```python
from build123d import *

# Parameters (mm, degrees)
THICKEN1_DEPTH      = 11.6
THICKEN1_START      = 10
THICKEN1_2_DEPTH    = 1.6
SKETCH2_R           = 1
BOSS_EXTRUDE1_DEPTH = 5
SKETCH3_W           = 9
SKETCH3_H           = 4
BOSS_EXTRUDE2_DEPTH = 4.5
CUT_EXTRUDE1_REACH  = 29.786
SKETCH4_RX          = 3.75
SKETCH4_RY          = 2.5
BOSS_EXTRUDE3_START = 7.5
BOSS_EXTRUDE3_DEPTH = 7.5
FILLET1_R           = 0.5
FILLET2_R           = 0.2


# Read off the part's stored shape, not the designer's step: Thicken1
with BuildPart() as part:
    # Thicken1 outline → Thicken1 (new body)
    with BuildSketch(Plane.XY):
        with BuildLine():
            Line((-8.73, -7.62), (8.73, -7.62))
            ThreePointArc((8.73, -7.62), (16.35, 0), (8.73, 7.62))
            Line((8.73, 7.62), (-8.73, 7.62))
            ThreePointArc((-8.73, 7.62), (-16.35, 0), (-8.73, -7.62))
        make_face()
        with BuildLine():
            ThreePointArc((8.73, 6.02), (14.75, 0), (8.73, -6.02))
            Line((8.73, -6.02), (-8.73, -6.02))
            ThreePointArc((-8.73, -6.02), (-14.75, 0), (-8.73, 6.02))
            Line((-8.73, 6.02), (8.73, 6.02))
        make_face(mode=Mode.SUBTRACT)
    extrude(amount=THICKEN1_DEPTH)

    # Thicken1 2 outline → Thicken1 2 (add)
    with BuildSketch(Plane.XY.offset(THICKEN1_START)):
        with BuildLine():
            Line((-8.73, -6.02), (8.73, -6.02))
            ThreePointArc((8.73, -6.02), (14.75, 0), (8.73, 6.02))
            Line((8.73, 6.02), (-8.73, 6.02))
            ThreePointArc((-8.73, 6.02), (-14.75, 0), (-8.73, -6.02))
        make_face()
    extrude(amount=THICKEN1_2_DEPTH)

    # Sketch2 → Boss-Extrude1 (add)
    with BuildSketch(Plane(origin=(0, 0, 10), x_dir=(-1, 0, 0), z_dir=(0, 0, -1))):
        with BuildLine():
            Line((1.6, 6.02), (-1.6, 6.02))
            Line((-1.6, 6.02), (-1.6, 2.537715508))
            ThreePointArc((-1.6, 2.537715508), (-2.537715508, -1.6), (1.6, -2.537715508))
            ThreePointArc((1.6, -2.537715508), (3, 0), (1.6, 2.537715508))
            Line((1.6, 2.537715508), (1.6, 6.02))
        make_face()
        Circle(SKETCH2_R, mode=Mode.SUBTRACT)
    extrude(amount=BOSS_EXTRUDE1_DEPTH)

    # Sketch3 → Boss-Extrude2 (add)
    with BuildSketch(Plane.XY.offset(11.6)):
        with Locations((0, -9.62)):
            Rectangle(SKETCH3_W, SKETCH3_H)
    extrude(amount=-BOSS_EXTRUDE2_DEPTH)

    # Cut-Extrude1: up to this face of the body (flat: up to its plane)
    cut_extrude1_end = Plane(part.part.faces().sort_by_distance((0, -6.02, 5))[0])
    # Sketch4 → Cut-Extrude1 (cut, up to the picked face)
    with BuildSketch(Plane.XZ.offset(11.62), mode=Mode.PRIVATE) as cut_extrude1_sk1:
        with Locations(Location((0, 7.1), (0, 0, 0))):
            Ellipse(SKETCH4_RX, SKETCH4_RY)
    cut_extrude1_tool1 = split(extrude(cut_extrude1_sk1.sketch, amount=-CUT_EXTRUDE1_REACH, mode=Mode.PRIVATE), bisect_by=cut_extrude1_end, keep=Keep.BOTH, mode=Mode.PRIVATE)
    add(cut_extrude1_tool1.solids().sort_by(Axis((0, -11.62, 7.1), (0, 1, 0)))[0], mode=Mode.SUBTRACT)

    # Sketch6 → Boss-Extrude3 (add)
    with BuildSketch(Plane(origin=(0, 0, 10), x_dir=(-1, 0, 0), z_dir=(0, 0, -1)).offset(BOSS_EXTRUDE3_START)):
        with BuildLine():
            Line((-12.421097398, -3.691097398), (-12.986782823, -4.256782823))
            ThreePointArc((-12.986782823, -4.256782823), (-14.75, 0), (-12.986782823, 4.256782823))
            Line((-12.986782823, 4.256782823), (-12.421097398, 3.691097398))
            ThreePointArc((-12.421097398, 3.691097398), (-13.95, 0), (-12.421097398, -3.691097398))
        make_face()
        with BuildLine():
            Line((12.986782823, -4.256782823), (12.421097398, -3.691097398))
            ThreePointArc((12.421097398, -3.691097398), (13.95, 0), (12.421097398, 3.691097398))
            Line((12.421097398, 3.691097398), (12.986782823, 4.256782823))
            ThreePointArc((12.986782823, 4.256782823), (14.75, 0), (12.986782823, -4.256782823))
        make_face()
    extrude(amount=-BOSS_EXTRUDE3_DEPTH)

    # Fillet1
    fillet1_edges = [part.edges().sort_by_distance(p)[0] for p in [
        (-4.5, -7.62, 9.35),
        (-4.5, -11.62, 9.35),
        (4.5, -7.62, 9.35),
        (4.5, -11.62, 9.35),
        (1.6, 2.537715508, 7.5),
        (1.6, 6.02, 7.5),
        (-1.6, 6.02, 7.5),
        (-1.6, 2.537715508, 7.5),
        (-12.986782823, -4.256782823, 6.25),
        (-12.986782823, 4.256782823, 6.25),
        (12.986782823, 4.256782823, 6.25),
        (12.986782823, -4.256782823, 6.25),
    ]]
    fillet(fillet1_edges, radius=FILLET1_R)

    # Fillet2
    fillet2_edges = [part.edges().sort_by_distance(p)[0] for p in [
        (12.421097398, -3.691097398, 6.25),
        (12.421097398, 3.691097398, 6.25),
        (-12.421097398, 3.691097398, 6.25),
        (-12.421097398, -3.691097398, 6.25),
    ]]
    fillet(fillet2_edges, radius=FILLET2_R)


solid = part.part
```
Work out the finished part from the listing and answer in its coordinate system (mm). A direction names the side the tool comes from. Coordinates: 2 decimals unless noted, no trailing zeros. Loops run counter-clockwise (first coordinate to the right, second up) from the corner with the lowest first, then second, coordinate; pieces in that order, holes last. Notation, with made-up numbers: (45, 67.25) - (70, 67.25) arc R26 cw to (70, 96.25) - close; hole circle Ø10 at (-24, 74). An arc over 180 degrees is marked (long way). Use a Markdown table: item, result.
Item 1: For faces 1 (the flat face through (4.5, -10, 9)), 2 (the flat face through (0, 0, 10)), 3 (the flat face through (0, 0, 11.6)), 4 (the flat face through (4, -10, 7.1)), 5 (the flat face through (-4.5, -10, 9)), determine the directions among +Z, -Z, +X, -X, +Y, -Y from which every point of the face is accessible in a straight line to the end or side of a thin tool.
Evaluation:
| item | result |
|---|---|
| face 1 | +Z, -Z, +X, -Y |
| face 2 | -Z |
| face 3 | +Z, +X, -X, +Y, -Y |
| face 4 | -Z, +X, -X, -Y |
| face 5 | +Z, -Z, -X, -Y |
Item 2: Given pin 1 Ø1 at (x, z) = (3, 5) entering from -Y; pin 2 Ø1 at (y, z) = (2, 3) entering from +X; pin 3 Ø1.4 at (y, z) = (4, 8.5) entering from +X, each flat-ended and moving along its own axis, determine where each tip first touches the part or whether it passes through.
Evaluation:
| item | result |
|---|---|
| pin 1 | stops at y = -7.62 |
| pin 2 | stops at x = 16.2 |
| pin 3 | stops at x = 15.6 |
Item 3: Find section A-A, the plane z = 1.75. Determine the outline of the cut face in (x, y), and give its area (3 significant figures).
Evaluation:
| item | result |
|---|---|
| outline | (-8.73, -7.62) - (8.73, -7.62) arc R7.62 ccw to (8.73, 7.62) - (-8.73, 7.62) arc R7.62 ccw to start; hole (-8.73, -6.02) - (8.73, -6.02) arc R6.02 ccw to (8.73, 6.02) - (-8.73, 6.02) arc R6.02 ccw to start |
| area | 124 mm2 |
Item 4: Consider probe 1 along Y at (x, z) = (0, 6.6); probe 2 along X at (y, z) = (2.75, 8); probe 3 along Y at (x, z) = (7, 2.25). Determine where each line is inside the solid, lowest interval first. Write a range as from..to.
Evaluation:
| item | result |
|---|---|
| probe 1 | y = -3..-1, 1..7.62 |
| probe 2 | x = -15.84..-13.17, -1.6..1.6, 13.17..15.84 |
| probe 3 | y = -7.62..-6.02, 6.02..7.62 |
Item 5: Find section C-C, the plane x = 6. Determine the outline of the cut face in (y, z).
Evaluation:
| item | result |
|---|---|
| outline | (-7.62, 0) - (-6.02, 0) - (-6.02, 10) - (6.02, 10) - (6.02, 0) - (7.62, 0) - (7.62, 11.6) - (-7.62, 11.6) - close |
Item 6: Find section B-B, the plane y = 0. Determine the outline of the cut face in (x, z), and give its area (3 significant figures).
Evaluation:
| item | result |
|---|---|
| outline | (-16.35, 0) - (-14.75, 0) - (-14.75, 2.5) - (-13.95, 2.5) - (-13.95, 10) - (-3, 10) - (-3, 5) - (-1, 5) - (-1, 10) - (1, 10) - (1, 5) - (3, 5) - (3, 10) - (13.95, 10) - (13.95, 2.5) - (14.75, 2.5) - (14.75, 0) - (16.35, 0) - (16.35, 11.6) - (-16.35, 11.6) - close |
| area | 116 mm2 |
Item 7: Find section D-D, the plane z = 3.5. Determine the outline of the cut face in (x, y).
Evaluation:
| item | result |
|---|---|
| outline | (-8.73, -7.62) - (8.73, -7.62) arc R7.62 ccw to (8.73, 7.62) - (-8.73, 7.62) arc R7.62 ccw to start; hole (-12.62, -3.89) arc R0.5 ccw to (-12.58, -4.62) arc R6.02 ccw to (-8.73, -6.02) - (8.73, -6.02) arc R6.02 ccw to (12.58, -4.62) arc R0.5 ccw to (12.62, -3.89) - (12.56, -3.83) arc R0.2 cw to (12.55, -3.55) arc R5.22 ccw to (12.55, 3.55) arc R0.2 cw to (12.56, 3.83) - (12.62, 3.89) arc R0.5 ccw to (12.58, 4.62) arc R6.02 ccw to (8.73, 6.02) - (-8.73, 6.02) arc R6.02 ccw to (-12.58, 4.62) arc R0.5 ccw to (-12.62, 3.89) - (-12.56, 3.83) arc R0.2 cw to (-12.55, 3.55) arc R5.22 ccw to (-12.55, -3.55) arc R0.2 cw to (-12.56, -3.83) - close |
Item 8: The mould has two halves that part along Y. Classify faces 6 (the flat face through (0, -7.62, 4)), 7 (the cylindrical face through (-16.35, 0.17, 5.72)), 8 (the flat face through (-4, -10, 7.1)), 9 (the flat face through (-14.1, -0.3, 2.5)): +Y half, -Y half, draft (parallel to the pull), parting line (faces both ways), or undercut.
Evaluation:
| item | result |
|---|---|
| face 6 | -Y half |
| face 7 | parting line |
| face 8 | draft |
| face 9 | undercut |
